```python
from build123d import *

# Parameters (mm, degrees)
TABFACEPLATESKETCH_W      = 27
TABFACEPLATESKETCH_H      = 44.45
TABFACEPLATEPAD_DEPTH     = 4
TABFLANGESKETCH_W         = 5
TABFLANGESKETCH_H         = 44.45
TABFLANGEPAD_DEPTH        = 14
BOTTOMGUSSETPAD_DEPTH     = 4
TOPGUSSETPAD_DEPTH        = 4
RAILHOLESSKETCH_R         = 2.3
RAILHOLESSKETCH_R_2       = 3.15
RAILHOLESPOCKET_DEPTH     = 18.001
TABJOINTHOLESSKETCH_R     = 1.6
TABJOINTHOLESPOCKET_DEPTH = 5.001
TABINSIDEFILLETS_R        = 2


with BuildPart() as part:
    # TabFacePlateSketch → TabFacePlatePad (new body)
    with BuildSketch(Plane.XY):
        with Locations((-13.5, 22.225)):
            Rectangle(TABFACEPLATESKETCH_W, TABFACEPLATESKETCH_H)
    extrude(amount=TABFACEPLATEPAD_DEPTH)

    # TabFlangeSketch (on Face6 of TabFacePlatePad) → TabFlangePad (join)
    with BuildSketch(Plane.XY.offset(4)):
        with Locations((-2.5, 22.225)):
            Rectangle(TABFLANGESKETCH_W, TABFLANGESKETCH_H)
    extrude(amount=TABFLANGEPAD_DEPTH)

    # BottomGussetSketch (on Face6 of TabFlangePad) → BottomGussetPad (join)
    with BuildSketch(Plane.XZ):
        Polygon((-12, 4), (-5, 4), (-5, 18), align=None)
    extrude(amount=-BOTTOMGUSSETPAD_DEPTH)

    # TopGussetSketch (on Face2 of BottomGussetPad) → TopGussetPad (join)
    with BuildSketch(Plane(origin=(0, 44.45, 0), x_dir=(-1, 0, 0), z_dir=(0, 1, 0))):
        Polygon((12, 4), (5, 4), (5, 18), align=None)
    extrude(amount=-TOPGUSSETPAD_DEPTH)

    # RailHolesSketch (on Face3 of TopGussetPad) → RailHolesPocket (cut, through all)
    with BuildSketch(Plane(origin=(0, 0, 0), x_dir=(1, 0, 0), z_dir=(0, 0, -1))):
        with Locations((-18, -6.225)):
            Circle(RAILHOLESSKETCH_R)
        with Locations((-18, -22.225)):
            Circle(RAILHOLESSKETCH_R_2)
        with Locations((-18, -38.225)):
            Circle(RAILHOLESSKETCH_R)
    extrude(amount=-RAILHOLESPOCKET_DEPTH, mode=Mode.SUBTRACT)

    # TabJointHolesSketch (on Face14 of RailHolesPocket) → TabJointHolesPocket (cut, through all)
    with BuildSketch(Plane(origin=(-5, 0, 0), x_dir=(0, -1, 0), z_dir=(-1, 0, 0))):
        with Locations((-11, 11)):
            Circle(TABJOINTHOLESSKETCH_R)
        with Locations((-33.45, 11)):
            Circle(TABJOINTHOLESSKETCH_R)
    extrude(amount=-TABJOINTHOLESPOCKET_DEPTH, mode=Mode.SUBTRACT)

    # TabInsideFillets
    tabinsidefillets_edges = [part.edges().sort_by_distance(p)[0] for p in [
        (-5, 22.225, 4),
        (-5, 40.45, 11),
        (-5, 4, 11),
        (-8.5, 40.45, 4),
        (-8.5, 4, 4),
    ]]
    fillet(tabinsidefillets_edges, radius=TABINSIDEFILLETS_R)


solid = part.part
```
Geometry check sheet. Reference: the model listing, model coordinates, mm. A direction names the side the tool comes from. Coordinates: 2 decimals unless noted, no trailing zeros. Order: outer loops, then holes, each group sorted by start corner. A loop starts at its lowest first (then second) coordinate and runs counter-clockwise, first axis right, second up.
Q1. Sectioned sample at A-A on y = 11. Record the cut outline in (x, z), and give its area (3 significant figures).
Reply:
outline: (-27, 0) - (0, 0) - (0, 9.4) - (-5, 9.4) - (-5, 6) arc R2 cw to (-7, 4) - (-27, 4) - close; (-5, 12.6) - (0, 12.6) - (0, 18) - (-5, 18) - close
area: 163 mm2
Q2. Sectioned sample at D-D on x = -2. Record the cut outline in (y, z), and give its area (3 significant figures).
Reply:
outline: (0, 0) - (44.45, 0) - (44.45, 18) - (0, 18) - close; hole circle Ø3.2 at (11, 11); hole circle Ø3.2 at (33.45, 11)
area: 784 mm2
Q3. Thickness scan on probe 1 along Y at (x, z) = (-18, 1) (3 decimals); probe 2 along Z at (x, y) = (-10.5, 15.5); probe 3 along X at (y, z) = (32, 15). Record the ranges inside material, lowest first.
Reply:
probe 1: y = 0 to 3.925, 8.525 to 19.075, 25.375 to 35.925, 40.525 to 44.45
probe 2: z = 0 to 4
probe 3: x = -5 to 0
Q4. Tool access check on faces 1 (the face through (-27, 22, 2)), 2 (the face through (-5.57, 4.6, 12.08)). Record the directions out of +Z, -Z, +X, -X, +Y, -Y that give a thin tool (end or side, any length) a straight path to the whole face; none if there is none.
Reply:
face 1: +Z, -Z, -X, +Y, -Y
face 2: +Z, -X
Q5. Depth check by flat-ended pin: pin 1 Ø3.5 at (y, z) = (18, 10) entering from -X; pin 2 Ø2.5 at (y, z) = (33.45, 11) entering from -X; pin 3 Ø6 at (x, y) = (-19.5, 29.5) entering from +Z. Enter the tip coordinate at first touch or a pass-through.
Reply:
pin 1: stops at x = -5
pin 2: passes through
pin 3: stops at z = 4
Q6. Sectioned sample at C-C on z = 11. Record the cut outline in (x, y), and give its area (3 significant figures).
Reply:
outline: (-8.5, 0) - (0, 0) - (0, 9.4) - (-5, 9.4) - (-5, 6) arc R2 cw to (-7, 4) - (-8.5, 4) - close; (-8.5, 40.45) - (-7, 40.45) arc R2 cw to (-5, 38.45) - (-5, 35.05) - (0, 35.05) - (0, 44.45) - (-8.5, 44.45) - close; (-5, 12.6) - (0, 12.6) - (0, 31.85) - (-5, 31.85) - close
area: 220 mm2
Q7. Sectioned sample at B-B on x = -18. Record the cut outline in (y, z) (3 decimals), and give its area (3 significant figures).
Reply:
outline: (0, 0) - (3.925, 0) - (3.925, 4) - (0, 4) - close; (8.525, 0) - (19.075, 0) - (19.075, 4) - (8.525, 4) - close; (25.375, 0) - (35.925, 0) - (35.925, 4) - (25.375, 4) - close; (40.525, 0) - (44.45, 0) - (44.45, 4) - (40.525, 4) - close
area: 116 mm2
Q8. Draft check along Z on faces 3 (the face through (-2.54, 12.6, 11.07)), 4 (the face through (-9.46, 39.85, 4.57)), 5 (the face through (-8, 4, 8)). Enter one of: released by +Z, released by -Z, zero draft, split by the parting line, or undercut.
Reply:
face 3: undercut
face 4: released by +Z
face 5: zero draft
